Can you work these out from the drawing? Everything is in mm from the part's minimum corner. A direction names the side the tool comes from. Give positions to 0.01 mm unless a question says otherwise; leave off trailing zeros. Order: outer loops, then holes, each group sorted by start corner. A loop starts at its lowest first (then second) coordinate and runs counter-clockwise, first axis right, second up. Notation, with made-up numbers: (76.25, -23) - (100.25, -23) arc R31 ccw to (100.25, 12) - close; hole circle Ø1 at (38, -26.75). An arc over 180 degrees is marked (long way). One line per question, with ' | ' between items.
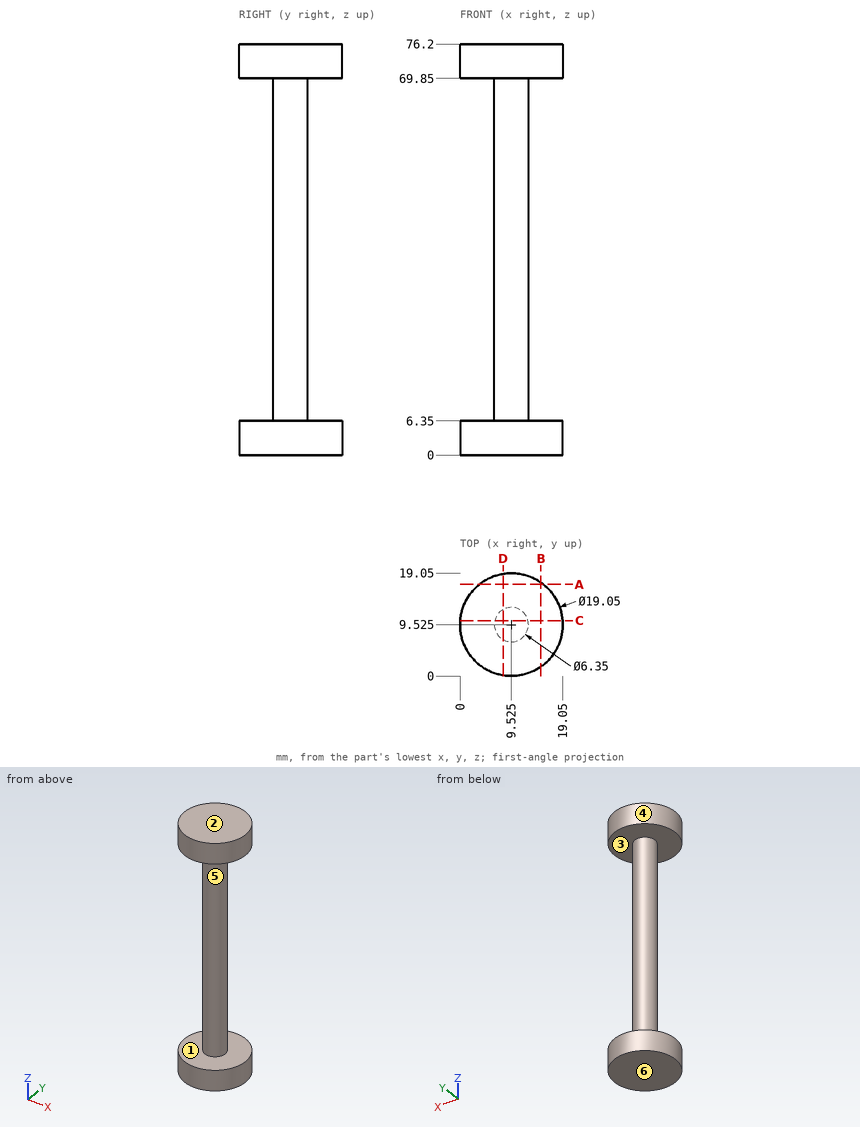
(1) On a 3-axis mill with a long thin cutter (end or side, diameter ignored), from which of +Z, -Z, +X, -X, +Y, -Y can I reach the whole of each face in a straight line? I mean the marked faces 1 and 2. Say none if no direction works.
Answer below:
face 1: none | face 2: +Z, +X, -X, +Y, -Y
(2) If we mould it in two halves opening along Z, with no side actions, what happens to the marked faces 3, 4, 5 and 6? For each: released by +Z, released by -Z, zero draft, split by the parting line, or undercut.
Answer below:
face 3: undercut | face 4: zero draft | face 5: undercut | face 6: released by -Z
(3) Imagine slicing it at B-B (x = 15). List the corners of the cut face in (y, z) for me, and give its area (3 significant figures).
Answer below:
outline: (1.73, 0) - (17.32, 0) - (17.32, 6.35) - (1.73, 6.35) - close; (1.73, 69.85) - (17.32, 69.85) - (17.32, 76.2) - (1.73, 76.2) - close | area: 198 mm^2
(4) If I drill on line 1 (Z direction, x = 13.75, y = 6); line 2 (X direction, y = 9.75, z = 43), over which ranges is the centre line in solid material (lowest first)?
Answer below:
line 1: 0 to 6.35, 69.85 to 76.2 | line 2: 6.36 to 12.69
(5) Imagine slicing it at D-D (x = 8). List the corners of the cut face in (y, z) for me, and give its area (3 significant figures).
Answer below:
outline: (0.12, 0) - (18.93, 0) - (18.93, 6.35) - (12.31, 6.35) - (12.31, 69.85) - (18.93, 69.85) - (18.93, 76.2) - (0.12, 76.2) - (0.12, 69.85) - (6.74, 69.85) - (6.74, 6.35) - (0.12, 6.35) - close | area: 592 mm^2
(6) Imagine slicing it at C-C (y = 10.25). List the corners of the cut face in (x, z) for me.
Answer below:
outline: (0.03, 0) - (19.02, 0) - (19.02, 6.35) - (12.62, 6.35) - (12.62, 69.85) - (19.02, 69.85) - (19.02, 76.2) - (0.03, 76.2) - (0.03, 69.85) - (6.43, 69.85) - (6.43, 6.35) - (0.03, 6.35) - close
(7) Will these pins go through, and if not, where does the flat tip stop? pin 1 (10 mm diameter, centred on y = 15.5, z = 40.5, fed in from +X); pin 2 (8 mm diameter, centred on x = 3, z = 29.5, fed in from +Y).
Answer below:
pin 1: x = 12.55 | pin 2: y = 11.45
(8) Imagine slicing it at A-A (y = 17). List the corners of the cut face in (x, z) for me.
Answer below:
outline: (3.62, 0) - (15.43, 0) - (15.43, 6.35) - (3.62, 6.35) - close; (3.62, 69.85) - (15.43, 69.85) - (15.43, 76.2) - (3.62, 76.2) - close
